Model file for the job. Use its own axes, mm. Give positions to 0.01 mm unless a question says otherwise; leave off trailing zeros. Answer in a Markdown table with one row per item.
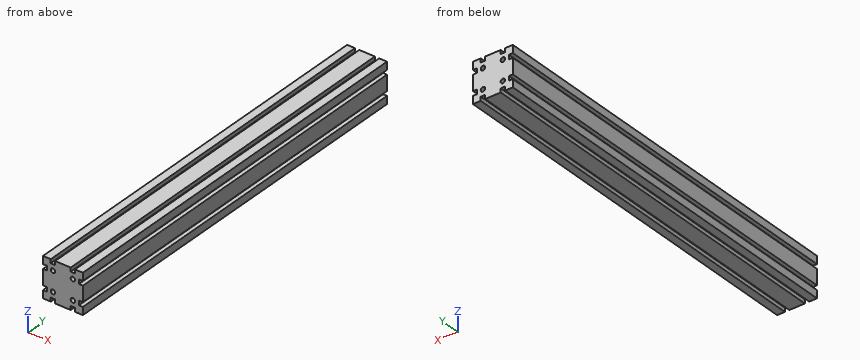
```python
from build123d import *

# Parameters (mm, degrees)
F0_R     = 5
F1_DEPTH = 881


with BuildPart() as f1:
    # F0 (on Front) → F1 (new body)
    with BuildSketch(Plane.XZ):
        Polygon((36.25, -45), (45, -45), (45, -27.5), (36.25, -27.5), (36.25, -17.5), (45, -17.5), (45, 17.5), (36.25, 17.5), (36.25, 27.5), (45, 27.5), (45, 45), (27.5, 45), (27.5, 36.25), (17.5, 36.25), (17.5, 45), (-17.5, 45), (-17.5, 36.25), (-27.5, 36.25), (-27.5, 45), (-45, 45), (-45, 27.5), (-36.25, 27.5), (-36.25, 17.5), (-45, 17.5), (-45, -17.5), (-36.25, -17.5), (-36.25, -27.5), (-45, -27.5), (-45, -45), (-27.5, -45), (-27.5, -36.25), (-17.5, -36.25), (-17.5, -45), (17.5, -45), (17.5, -36.25), (27.5, -36.25), (27.5, -45), align=None)
        with Locations((-22.5, -22.5)):
            Circle(F0_R, mode=Mode.SUBTRACT)
        with Locations((22.5, -22.5)):
            Circle(F0_R, mode=Mode.SUBTRACT)
        with Locations((-22.5, 22.5)):
            Circle(F0_R, mode=Mode.SUBTRACT)
        with Locations((22.5, 22.5)):
            Circle(F0_R, mode=Mode.SUBTRACT)
    extrude(amount=F1_DEPTH)


solid = f1.part
```
Q1. Probe probe 1 along Z at (x, y) = (38, -131.5); probe 2 along X at (y, z) = (-307, -22); probe 3 along Z at (x, y) = (22.5, -508). List the from-to ranges inside material, lowest first.
Reported:
| item | result |
|---|---|
| probe 1 | -45 to -27.5, -17.5 to 17.5, 27.5 to 45 |
| probe 2 | -36.25 to -27.47, -17.53 to 17.53, 27.47 to 36.25 |
| probe 3 | -36.25 to -27.5, -17.5 to 17.5, 27.5 to 36.25 |
Q2. Drop flat-ended pins along their axis: pin 1 (9 mm diameter, centred on x = -22.5, z = 22.5, fed in from +Y); pin 2 (5 mm diameter, centred on y = -584.5, z = 24, fed in from -X); pin 3 (5 mm diameter, centred on y = -250.5, z = -24, fed in from +X). Give the stop position or say it passes through.
Reported:
| item | result |
|---|---|
| pin 1 | through |
| pin 2 | x = -36.25 |
| pin 3 | x = 36.25 |
Q3. Saw through at A-A (y = -283). Give the number of separate pieces and of enclosed holes in the cut face, and give its area (3 significant figures).
Reported:
| item | result |
|---|---|
| separate pieces | 1 |
| enclosed holes | 4 |
| area | 7,090 mm² |
